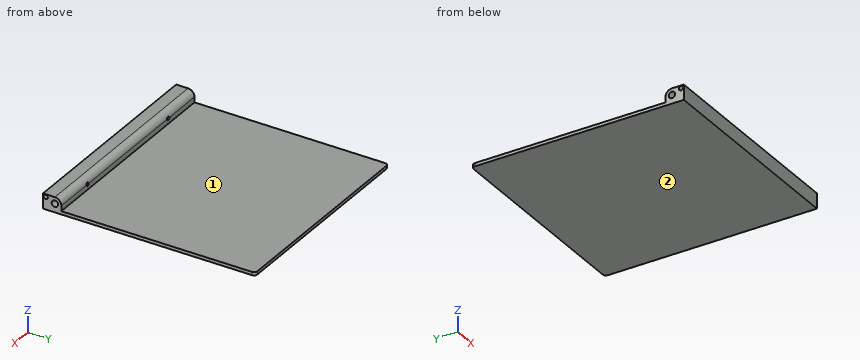
```python
from build123d import *

# Parameters (mm, degrees)
SKETCH1_W           = 198
SKETCH1_H           = 180
BOSS_EXTRUDE1_DEPTH = 3
SKETCH3_R           = 3
BOSS_EXTRUDE2_DEPTH = 198
SKETCH12_R          = 1.65
CUT_EXTRUDE1_DEPTH  = 5
SKETCH4_W           = 198
SKETCH4_H           = 3
BOSS_EXTRUDE3_DEPTH = 17
SKETCH10_W          = 198
SKETCH10_H          = 2
BOSS_EXTRUDE7_DEPTH = 10
FILLET2_R           = 3
BOSS_EXTRUDE8_DEPTH = 198
SKETCH15_R          = 2
CUT_EXTRUDE4_DEPTH  = 4


with BuildPart() as part:
    # Sketch1 → Boss-Extrude1 (new body)
    with BuildSketch(Plane.XY):
        with Locations((99, 90)):
            Rectangle(SKETCH1_W, SKETCH1_H)
    extrude(amount=BOSS_EXTRUDE1_DEPTH)

    # Sketch3 → Boss-Extrude2 (add)
    with BuildSketch(Plane.ZY):
        with BuildLine():
            Line((0, 0), (8, 0))
            ThreePointArc((8, 0), (14, -6), (8, -12))
            Line((8, -12), (0, -12))
            Line((0, -12), (0, 0))
        make_face()
        with Locations((8, -6)):
            Circle(SKETCH3_R, mode=Mode.SUBTRACT)
    extrude(amount=-BOSS_EXTRUDE2_DEPTH)

    # Sketch12 → Cut-Extrude1 (cut)
    with BuildSketch(Plane(origin=(0, 0, 0), x_dir=(1, 0, 0), z_dir=(0, 1, 0))):
        with Locations((39, -8)):
            Circle(SKETCH12_R)
        with Locations((159, -8)):
            Circle(SKETCH12_R)
    extrude(amount=-CUT_EXTRUDE1_DEPTH, mode=Mode.SUBTRACT)

    # Sketch4 → Boss-Extrude3 (add)
    with BuildSketch(Plane.XZ):
        with Locations((99, 1.5)):
            Rectangle(SKETCH4_W, SKETCH4_H)
    extrude(amount=BOSS_EXTRUDE3_DEPTH)

    # Sketch10 → Boss-Extrude7 (add)
    with BuildSketch(Plane.XY.offset(3)):
        with Locations((99, -16)):
            Rectangle(SKETCH10_W, SKETCH10_H)
    extrude(amount=BOSS_EXTRUDE7_DEPTH)

    # Fillet2
    fillet2_edges = [part.edges().sort_by_distance(p)[0] for p in [
        (198, 180, 1.5),
        (0, 180, 1.5),
        (0, -17, 6.5),
        (198, -17, 6.5),
    ]]
    fillet(fillet2_edges, radius=FILLET2_R)

    # Sketch11 → Boss-Extrude8 (add)
    with BuildSketch(Plane.ZY):
        with BuildLine():
            Line((11, -6), (14, -6))
            Line((14, -6), (14, -17))
            Line((14, -17), (0, -17))
            Line((0, -17), (0, -6))
            Line((0, -6), (5, -6))
            ThreePointArc((5, -6), (8, -9), (11, -6))
        make_face()
    extrude(amount=-BOSS_EXTRUDE8_DEPTH)

    # Sketch15 → Cut-Extrude4 (cut)
    with BuildSketch(Plane(origin=(198, 0, 0), x_dir=(0, 0, -1), z_dir=(1, 0, 0))):
        with Locations((-11.5, -14.5)):
            Circle(SKETCH15_R)
    cut_extrude4 = extrude(amount=-CUT_EXTRUDE4_DEPTH, mode=Mode.SUBTRACT)

    # Mirror3: Cut-Extrude4 across plane
    add(cut_extrude4.mirror(Plane.ZY.offset(-99)), mode=Mode.SUBTRACT)


solid = part.part
```
The model under review builds one solid part; all positions refer to its coordinate system, in mm. Face numbers are marked on the shaded views. A direction names the side the tool comes from. Coordinates: 2 decimals unless noted, no trailing zeros. Loops run counter-clockwise (first coordinate to the right, second up) from the corner with the lowest first, then second, coordinate; pieces in that order, holes last. Notation, with made-up numbers: (16, -18.5) -> (28, -18.5) arc R29 cw to (28, 18.5) -> close; hole circle Ø2 at (84, 0.25). An arc over 180 degrees is marked (long way). Answer as CSV lines item,"result".
Item 1: Machinability: for the marked faces 1 and 2, which of the approach directions +Z, -Z, +X, -X, +Y, -Y give a long, thin tool a straight path to every point of the face, cutting with its end or side? Answer none if there is none.
Results below:
face 1,"+Z, +X, -X, +Y"
face 2,"-Z, +X, -X, +Y, -Y"
Item 2: For L1, parallel to X at y = -2.2, z = 8; L2, parallel to Y at x = 131.5, z = 8.5; L3, parallel to Y at x = 67.5, z = 3.25, list the stretches that pass through material, from the lowest coordinate up.
Results below:
L1,"x = 0 to 37.35, 40.65 to 157.35, 160.65 to 198"
L2,"y = -17 to -8.96, -3.04 to -0.02"
L3,"y = -17 to 0"
Item 3: Take a section at A-A, the plane x = 167.5. State the section outline as (y, z) points.
Results below:
outline,"(-17, 0) -> (180, 0) -> (180, 3) -> (0, 3) -> (0, 8) arc R6 ccw to (-6, 14) -> (-17, 14) -> close; hole circle Ø6 at (-6, 8)"
Item 4: Insertion check: pin 1 (2.5 mm diameter, centred on x = 96, z = 4.5, fed in from +Y); pin 2 (5 mm diameter, centred on x = 62, y = 131.5, fed in from +Z); pin 3 (1.2 mm diameter, centred on y = -14, z = 12.5, fed in from +X). Each pin has a flat end and moves straight along its axis. Give the tip position at first contact, or say it passes through.
Results below:
pin 1,"stops at y = 0"
pin 2,"stops at z = 3"
pin 3,"stops at x = 194"
Item 5: Take a section at B-B, the plane y = 109.5. State the section outline as (x, z) points, and give its area (3 significant figures).
Results below:
outline,"(0, 0) -> (198, 0) -> (198, 3) -> (0, 3) -> close"
area,"594 mm2"
